from build123d import *

# Parameters (mm, degrees)
SKETCH1_W           = 127
SKETCH1_H           = 90
BOSS_EXTRUDE1_DEPTH = 228
SKETCH2_R           = 6.5
CUT_EXTRUDE1_DEPTH  = 228
SKETCH3_W           = 127
SKETCH3_H           = 228
SKETCH3_R           = 6.5
BOSS_EXTRUDE2_DEPTH = 18


with BuildPart() as part:
    # Sketch1 → Boss-Extrude1 (new body)
    with BuildSketch(Plane.XY):
        Rectangle(SKETCH1_W, SKETCH1_H)
    extrude(amount=BOSS_EXTRUDE1_DEPTH)

    # Sketch2 → Cut-Extrude1 (cut)
    with BuildSketch(Plane(origin=(0, 45, 0), x_dir=(1, 0, 0), z_dir=(0, 1, 0))):
        with Locations((-39.802347905, -28.441961554)):
            Circle(SKETCH2_R)
        with Locations((41.843493952, -208.06281364)):
            Circle(SKETCH2_R)
    extrude(amount=-CUT_EXTRUDE1_DEPTH, mode=Mode.SUBTRACT)

    # Sketch3 → Boss-Extrude2 (add)
    with BuildSketch(Plane(origin=(0, 45, 0), x_dir=(1, 0, 0), z_dir=(0, 1, 0))):
        with Locations((0, -114)):
            Rectangle(SKETCH3_W, SKETCH3_H)
        with Locations((-39.802347905, -28.441961554)):
            Circle(SKETCH3_R, mode=Mode.SUBTRACT)
        with Locations((41.843493952, -208.06281364)):
            Circle(SKETCH3_R, mode=Mode.SUBTRACT)
    extrude(amount=BOSS_EXTRUDE2_DEPTH)


solid = part.part
Design review of the part built by this model. Coordinates are the model's own, in mm. Round coordinates to 2 decimals unless told otherwise and drop trailing zeros. Loops run counter-clockwise (first coordinate to the right, second up) from the corner with the lowest first, then second, coordinate; pieces in that order, holes last. Notation, with made-up numbers: (27, 72.25) -> (65, 72.25) arc R15 ccw to (65, 96.25) -> close; hole circle Ø4 at (61, 57.25). An arc over 180 degrees is marked (long way). Use one line per item in the form item = value. Start each with the question number.
Q1. Wall thickness on line 1 along Z through (x, y) = (42.5, -17); line 2 along Z through (x, y) = (-40, 18): over which ranges is each line inside the solid? List them lowest first. Write a range as [from, to].
Q2. We need section B-B on x = 41. Give the boundary of the cut face in (y, z).
Q3. For pin 1 Ø8 at (x, z) = (41.84, 208.06) entering from +Y; pin 2 Ø4 at (x, y) = (19.5, 50) entering from -Z, all flat-tipped, find the tip position at first contact; note any pin that passes through.
Q4. We need section A-A on x = -39.5. Give the boundary of the cut face in (y, z).
Calculated:
q1.line_1 = [0, 201.6], [214.53, 228]
q1.line_2 = [0, 21.94], [34.94, 228]
q2.outline = (-45, 0) -> (63, 0) -> (63, 201.62) -> (-45, 201.62) -> close; (-45, 214.51) -> (63, 214.51) -> (63, 228) -> (-45, 228) -> close
q3.pin_1 = through
q3.pin_2 = 0
q4.outline = (-45, 0) -> (63, 0) -> (63, 21.95) -> (-45, 21.95) -> close; (-45, 34.93) -> (63, 34.93) -> (63, 228) -> (-45, 228) -> close
